Check sheet for the modelled part. Datum: model origin and axes. Units: mm. Give positions to 0.01 mm unless a question says otherwise; leave off trailing zeros. Order: outer loops, then holes, each group sorted by start corner. A loop starts at its lowest first (then second) coordinate and runs counter-clockwise, first axis right, second up. Notation, with made-up numbers: M 12.25,33 L 40.25,33 A19 cw 40.25,52 Z; hole C -11,86.5 d4. An arc over 180 degrees is marked long. Answer in a Markdown table with one row per item. Add a question column.
from build123d import *

# Parameters (mm, degrees)
SKETCH1_R           = 75
SKETCH1_R_2         = 1.75
SKETCH1_R_3         = 6
BOSS_EXTRUDE1_DEPTH = 5
CUT_EXTRUDE1_DEPTH  = 107.183802908


with BuildPart() as part:
    # Sketch1 → Boss-Extrude1 (new body)
    with BuildSketch(Plane(origin=(0, 0, 0), x_dir=(1, 0, 0), z_dir=(0, 1, 0))):
        with Locations(Location((0, 0, 0), (0, 0, 270))):
            Circle(SKETCH1_R)
        with Locations(Location((32, 0, 0), (0, 0, 270))):
            Circle(SKETCH1_R_2, mode=Mode.SUBTRACT)
        with Locations(Location((0, 0, 0), (0, 0, 270))):
            Circle(SKETCH1_R_3, mode=Mode.SUBTRACT)
        Polygon((3.464101615, -51), (6.92820323, -45), (3.464101615, -39), (-3.464101615, -39), (-6.92820323, -45), (-3.464101615, -51), align=None, mode=Mode.SUBTRACT)
    extrude(amount=BOSS_EXTRUDE1_DEPTH)

    # Sketch2 → Cut-Extrude1 (cut, through all)
    with BuildSketch(Plane(origin=(0, 5, 0), x_dir=(1, 0, 0), z_dir=(0, 1, 0))):
        with BuildLine():
            Line((-45.916707554, 46.007129527), (-5, 10))
            Line((-5, 10), (0, 10))
            Line((0, 10), (0, 65))
            ThreePointArc((0, 65), (-24.844884591, 60.064396356), (-45.916707554, 46.007129527))
        make_face()
        with BuildLine():
            Line((-46.904157598, -45), (-15, 0))
            Line((-15, 0), (-54.772255751, 35))
            ThreePointArc((-54.772255751, 35), (-64.687891122, -6.362133458), (-46.904157598, -45))
        make_face()
        with BuildLine():
            Line((20, 61.846584384), (20, 10))
            Line((20, 10), (32, 10))
            Line((32, 10), (51.23475383, 40))
            ThreePointArc((51.23475383, 40), (37.254742659, 53.264285871), (20, 61.846584384))
        make_face()
        with BuildLine():
            Line((-15, -24.104744769), (-36.190322049, -53.993153177))
            ThreePointArc((-36.190322049, -53.993153177), (-26.00988263, -59.569169925), (-15, -63.245553203))
            Line((-15, -63.245553203), (-15, -24.104744769))
        make_face()
        with BuildLine():
            Line((32, -10), (15, -10))
            Line((15, -10), (15, -63.245553203))
            ThreePointArc((15, -63.245553203), (33.63849917, -55.618804137), (49.048013306, -42.653163901))
            Line((49.048013306, -42.653163901), (32, -10))
        make_face()
        with BuildLine():
            Line((59.203473805, 26.831859597), (42, 0))
            Line((42, 0), (57.662812973, -30))
            ThreePointArc((57.662812973, -30), (64.976128791, -1.761444678), (59.203473805, 26.831859597))
        make_face()
    extrude(amount=-CUT_EXTRUDE1_DEPTH, mode=Mode.SUBTRACT)


solid = part.part
Q1. Thickness scan on probe 1 along X at (y, z) = (3.3, 0); probe 2 along X at (y, z) = (3.15, 17); probe 3 along X at (y, z) = (0.9, -52). Record the ranges inside material, lowest first.
Q2. Cross-section at B-B (y = 4). State how many separate pieces and enclosed holes the cut face has, and give its area (3 significant figures).
Q3. Cross-section at A-A (z = 18.5). Record the boundary of the cut face in (x, y), and give its area (3 significant figures).
Q4. Draft check along Z on faces 1 (the flat face through (-15.6, 0, -1.1)), 2 (the flat face through (0, 2, 51)). Enter one of: pulls with the +Z half, pulls with the -Z half, needs draft (parallel to the pull), parting line crosses it, or undercut.
Q5. Go/stop test with flat-tipped pins: pin 1 (1.5 mm diameter, centred on x = -3.5, y = 3, fed in from -Z); pin 2 (1.5 mm diameter, centred on x = -16, y = 2, fed in from -Z); pin 3 (2.5 mm diameter, centred on x = 28, y = 1.5, fed in from -Z); pin 4 (3 mm diameter, centred on x = 32, z = 0, fed in from +Y). Record where each tip stops, or that it passes through.
Q6. Cross-section at D-D (x = -11). Record the boundary of the cut face in (y, z).
Q7. Cross-section at C-C (x = 22.5). Record the boundary of the cut face in (y, z).
Values follow:
| question | item | result |
|---|---|---|
| 1 | probe 1 | -75 to -65, -15 to -6, 6 to 30.25, 33.75 to 42, 65 to 75 |
| 1 | probe 2 | -73.05 to -62.74, -27.05 to 15, 35.65 to 50.88, 62.74 to 73.05 |
| 1 | probe 3 | -54.05 to -39, 0 to 20, 39 to 54.05 |
| 2 | separate pieces | 1 |
| 2 | enclosed holes | 9 |
| 2 | area | 10,200 mm² |
| 3 | outline | M -72.68,0 L -62.31,0 L -62.31,5 L -72.68,5 Z; M -28.12,0 L 15,0 L 15,5 L -28.12,5 Z; M 36.44,0 L 51.66,0 L 51.66,5 L 36.44,5 Z; M 62.31,0 L 72.68,0 L 72.68,5 L 62.31,5 Z |
| 3 | area | 395 mm² |
| 4 | face 1 | needs draft |
| 4 | face 2 | undercut |
| 5 | pin 1 | z = -74.95 |
| 5 | pin 2 | z = -73.43 |
| 5 | pin 3 | z = -70.07 |
| 5 | pin 4 | through |
| 6 | outline | M 0,-74.19 L 5,-74.19 L 5,-64.06 L 0,-64.06 Z; M 0,-15.28 L 5,-15.28 L 5,74.19 L 0,74.19 Z |
| 7 | outline | M 0,-71.55 L 5,-71.55 L 5,-60.98 L 0,-60.98 Z; M 0,-10 L 5,-10 L 5,10 L 0,10 Z; M 0,60.98 L 5,60.98 L 5,71.55 L 0,71.55 Z |
